The model under review builds one solid part; all positions refer to its coordinate system, in mm. Face numbers are marked on the shaded views. A direction names the side the tool comes from. Give positions to 0.01 mm unless a question says otherwise; leave off trailing zeros. Loops run counter-clockwise (first coordinate to the right, second up) from the corner with the lowest first, then second, coordinate; pieces in that order, holes last. Notation, with made-up numbers: (0.5, 21) - (57.5, 21) arc R21 ccw to (57.5, 53) - close; hole circle Ø1 at (44.25, 65). An arc over 180 degrees is marked (long way). Answer as a JSON object with one key per item and string values.
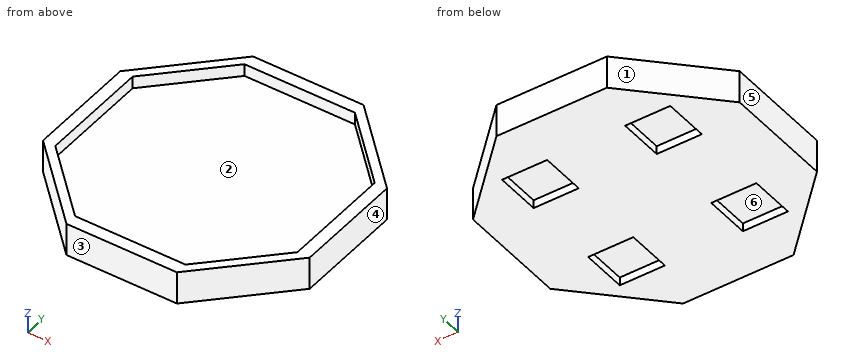
from build123d import *

# Parameters (mm, degrees)
F1_DEPTH = 5
F2_W     = 3
F2_H     = 26.923882
F2_W_2   = 26.923882
F2_H_2   = 3
F3_DEPTH = 3
F4_W     = 11
F4_H     = 11
F5_DEPTH = 2


with BuildPart() as f1:
    # F0 (on Top) → F1 (new body)
    with BuildSketch(Plane.XY):
        Polygon((-13.461941, -32.5), (13.461941, -32.5), (32.5, -13.461941), (32.5, 13.461941), (13.461941, 32.5), (-13.461941, 32.5), (-32.5, 13.461941), (-32.5, -13.461941), align=None)
    extrude(amount=F1_DEPTH)

    # F2 (on face) → F3 (join)
    with BuildSketch(Plane.XY.offset(5)):
        Polygon((-13.461941, 32.5), (-32.5, 13.461941), (-29.5, 13.461941), (-13.461941, 29.5), (13.461941, 29.5), (29.5, 13.461941), (29.5, -13.461941), (32.5, -13.461941), (32.5, 13.461941), (13.461941, 32.5), align=None)
        with Locations((-31, 0)):
            Rectangle(F2_W, F2_H)
        Polygon((-29.5, -13.461941), (-32.5, -13.461941), (-13.461941, -32.5), (-13.461941, -29.5), align=None)
        with Locations((0, -31)):
            Rectangle(F2_W_2, F2_H_2)
        Polygon((13.461941, -29.5), (13.461941, -32.5), (32.5, -13.461941), (29.5, -13.461941), align=None)
    extrude(amount=F3_DEPTH)

    # F4 (on face) → F5 (cut)
    with BuildSketch(Plane(origin=(0, 0, 0), x_dir=(1, 0, 0), z_dir=(0, 0, -1))):
        with Locations((-15, 15)):
            Rectangle(F4_W, F4_H)
        with Locations((15, 15)):
            Rectangle(F4_W, F4_H)
        with Locations((15, -15)):
            Rectangle(F4_W, F4_H)
        with Locations((-15, -15)):
            Rectangle(F4_W, F4_H)
    extrude(amount=-F5_DEPTH, mode=Mode.SUBTRACT)


solid = f1.part
Q1. Consider section C-C, the plane y = -19.5. State the section outline as (x, z) points, plus the area to 3 significant figures.
Results:
{"outline": "(-26.46, 0) - (-20.5, 0) - (-20.5, 2) - (-9.5, 2) - (-9.5, 0) - (9.5, 0) - (9.5, 2) - (20.5, 2) - (20.5, 0) - (26.46, 0) - (26.46, 8) - (23.46, 8) - (23.46, 5) - (-23.46, 5) - (-23.46, 8) - (-26.46, 8) - close", "area": "239 mm^2"}
Q2. The part is to be moulded in two halves that separate along Y. For the marked faces 1, 2, 3 and 4, say which applies: +Y half, -Y half, draft (parallel to the pull), parting line (faces both ways), or undercut.
Results:
{"face 1": "+Y half", "face 2": "undercut", "face 3": "-Y half", "face 4": "draft"}
Q3. Consider section A-A, the plane x = 6. State the section outline as (y, z) points.
Results:
{"outline": "(-32.5, 0) - (32.5, 0) - (32.5, 8) - (29.5, 8) - (29.5, 5) - (-29.5, 5) - (-29.5, 8) - (-32.5, 8) - close"}
Q4. Consider section B-B, the plane z = 4. State the section outline as (x, y) points, plus the area to 3 significant figures.
Results:
{"outline": "(-32.5, -13.46) - (-13.46, -32.5) - (13.46, -32.5) - (32.5, -13.46) - (32.5, 13.46) - (13.46, 32.5) - (-13.46, 32.5) - (-32.5, 13.46) - close", "area": "3,500 mm^2"}
Q5. Consider section D-D, the plane x = 16.5. State the section outline as (y, z) points.
Results:
{"outline": "(-29.46, 0) - (-20.5, 0) - (-20.5, 2) - (-9.5, 2) - (-9.5, 0) - (9.5, 0) - (9.5, 2) - (20.5, 2) - (20.5, 0) - (29.46, 0) - (29.46, 8) - (26.46, 8) - (26.46, 5) - (-26.46, 5) - (-26.46, 8) - (-29.46, 8) - close"}
Q6. Clearance check with flat-ended pins moving along their axes: pin 1 Ø0.6 at (y, z) = (-15.5, 1) entering from -X; pin 2 Ø8 at (x, y) = (-2, 25) entering from +Z; pin 3 Ø1 at (x, z) = (25.5, 1) entering from +Y. State where each tip first meets the part, or that it passes through.
Results:
{"pin 1": "stops at x = -30.76", "pin 2": "stops at z = 5", "pin 3": "stops at y = 20.96"}
Q7. To check wall thickness, follow probe 1 along Y at (x, z) = (-13, 1.5); probe 2 along Y at (x, z) = (-7, 6.75); probe 3 along Z at (x, y) = (-26, 6.5). State the ranges of each line that lie inside material, in increasing order. Write a range as [from, to].
Results:
{"probe 1": "y = [-32.5, -20.5], [-9.5, 9.5], [20.5, 32.5]", "probe 2": "y = [-32.5, -29.5], [29.5, 32.5]", "probe 3": "z = [0, 5]"}
Q8. For the marked faces 5 and 6, list the 3-axis set-ups (+Z, -Z, +X, -X, +Y, -Y) from which the entire face can be reached by the end or side of a thin tool; tool diameter is ignored.
Results:
{"face 5": "+Z, -Z, -X, +Y, -Y", "face 6": "-Z"}
